from build123d import *

# Parameters (mm, degrees)
F0_W     = 76.2
F0_H     = 43.18
F1_DEPTH = 25.4
F2_W     = 50.8
F2_H     = 6.35
F3_DEPTH = 43.181
F5_DEPTH = 12.7


with BuildPart() as f1:
    # F0 (on Top) → F1 (new body)
    with BuildSketch(Plane.XY):
        with Locations((34.672838, -9.800495)):
            Rectangle(F0_W, F0_H)
    extrude(amount=F1_DEPTH)

    # F2 (on face) → F3 (cut, through all)
    with BuildSketch(Plane.XZ.offset(31.390495)):
        with Locations((47.372838, 22.225)):
            Rectangle(F2_W, F2_H)
    extrude(amount=-F3_DEPTH, mode=Mode.SUBTRACT)

    # F4 (on face) → F5 (cut)
    with BuildSketch(Plane.XY.offset(19.05)):
        Polygon((39.164659, -1.706043), (21.972838, -1.706043), (21.972838, -18.966546), (39.164659, -18.966546), (39.164659, -31.390495), (72.772838, -31.390495), (72.772838, 11.789505), (39.164659, 11.789505), align=None)
    extrude(amount=-F5_DEPTH, mode=Mode.SUBTRACT)


solid = f1.part
Input: part model. Units: mm. Frame: model coordinates. A direction names the side the tool comes from. Round coordinates to 2 decimals unless told otherwise and drop trailing zeros. Order: outer loops, then holes, each group sorted by start corner. A loop starts at its lowest first (then second) coordinate and runs counter-clockwise, first axis right, second up. Notation, with made-up numbers: (23, 83) - (60, 83) arc R7 cw to (60, 94) - close; hole circle Ø6 at (-32.75, -13.75). An arc over 180 degrees is marked (long way). Use a Markdown table: item, result.
1. First-contact query: pin 1 (4 mm diameter, centred on y = -27, z = 10, fed in from +X); pin 2 (11 mm diameter, centred on x = 29.5, y = 3.5, fed in from +Z); pin 3 (1.5 mm diameter, centred on x = 62.5, z = 7, fed in from -Y); pin 4 (10 mm diameter, centred on x = 37, y = -9, fed in from +Z). Flat tips, straight axial feed; report the tip coordinate or a pass-through.
Evaluation:
| item | result |
|---|---|
| pin 1 | x = 39.16 |
| pin 2 | z = 19.05 |
| pin 3 | y = -31.39 |
| pin 4 | z = 6.35 |
2. Section C-C on y = -13.5. Return the cut outline in (x, z).
Evaluation:
| item | result |
|---|---|
| outline | (-3.43, 0) - (72.77, 0) - (72.77, 6.35) - (21.97, 6.35) - (21.97, 25.4) - (-3.43, 25.4) - close |
3. Mould query, pull axis Y, two halves, no side actions, for faces 4 (the face through (31, -1.706, 13)), 5 (the face through (26, -31.39, 10)), 6 (the face through (30, 5, 19.05)). Classes: +Y half, -Y half, draft (parallel to the pull), parting line (faces both ways), or undercut.
Evaluation:
| item | result |
|---|---|
| face 4 | undercut |
| face 5 | -Y half |
| face 6 | draft |
4. Section B-B on y = -26.5. Return the cut outline in (x, z), then the cut area to 3 significant figures.
Evaluation:
| item | result |
|---|---|
| outline | (-3.43, 0) - (72.77, 0) - (72.77, 6.35) - (39.16, 6.35) - (39.16, 19.05) - (21.97, 19.05) - (21.97, 25.4) - (-3.43, 25.4) - close |
| area | 1,190 mm^2 |
5. Section A-A on x = 26.5. Return the cut outline in (y, z), then the cut area to 3 significant figures.
Evaluation:
| item | result |
|---|---|
| outline | (-31.39, 0) - (11.79, 0) - (11.79, 19.05) - (-1.71, 19.05) - (-1.71, 6.35) - (-18.97, 6.35) - (-18.97, 19.05) - (-31.39, 19.05) - close |
| area | 603 mm^2 |
6. Section D-D on x = 61. Return the cut outline in (y, z), then the cut area to 3 significant figures.
Evaluation:
| item | result |
|---|---|
| outline | (-31.39, 0) - (11.79, 0) - (11.79, 6.35) - (-31.39, 6.35) - close |
| area | 274 mm^2 |
7. Access query for faces 1 (the face through (39.165, -25, 13)), 2 (the face through (26, 11.79, 10)), 3 (the face through (30, -18.967, 13)). Directions: +Z, -Z, +X, -X, +Y, -Y. A direction counts if a zero-diameter tool reaches every point of the face in a straight line with its end or side. Return the directions, or none.
Evaluation:
| item | result |
|---|---|
| face 1 | +Z, +X, +Y, -Y |
| face 2 | +Z, -Z, +X, -X, +Y |
| face 3 | +Z, +X |
8. Material intervals for probe 1 along Z at (x, y) = (32, -10.5); probe 2 along X at (y, z) = (-27.5, 15); probe 3 along Y at (x, z) = (23, 14.25), sorted ascending.
Evaluation:
| item | result |
|---|---|
| probe 1 | 0 to 6.35 |
| probe 2 | -3.43 to 39.16 |
| probe 3 | -31.39 to -18.97, -1.71 to 11.79 |
